from build123d import *

# Parameters (mm, degrees)
SKETCH_1_W                  = 40.6
SKETCH_1_H                  = 45
EXTRUDE_1_DEPTH             = 20
HOLE_WIZARD_M2_1_AT_2_COUNT = 2
HOLE_WIZARD_M2_1_AT_2_PITCH = 20


with BuildPart() as part:
    # 草图1 → 凸台-拉伸1 (new body)
    with BuildSketch(Plane(origin=(0, 0, 0), x_dir=(1, 0, 0), z_dir=(0, 1, 0))):
        Rectangle(SKETCH_1_W, SKETCH_1_H)
    extrude(amount=EXTRUDE_1_DEPTH)

    # 草图3 → M2 螺纹孔的螺纹孔钻头1 (revolve, cut)
    with BuildSketch(Plane(origin=(20.3, 10, 10), x_dir=(0, 0, -1), z_dir=(0, 1, 0))):
        Polygon((0, 0), (0, 8.480688495), (0.8, 8), (0.8, 0), align=None)
    hole_wizard_m2_1 = revolve(axis=Axis((26.65, 10, 10), (-1, 0, 0)), mode=Mode.SUBTRACT)

    # M2 螺纹孔的螺纹孔钻头1 at 2: M2 螺纹孔的螺纹孔钻头1 ×2
    with Locations(*[(0, 0, -i * HOLE_WIZARD_M2_1_AT_2_PITCH) for i in range(1, HOLE_WIZARD_M2_1_AT_2_COUNT)]):
        add(hole_wizard_m2_1, mode=Mode.SUBTRACT)

    # 镜向1: M2 螺纹孔的螺纹孔钻头1 across plane
    add(hole_wizard_m2_1.mirror(Plane(origin=(0, 0, 0), x_dir=(0, 0, 1), z_dir=(1, 0, 0))), mode=Mode.SUBTRACT)

    # 镜向1 copy 1 sketch → 镜向1 copy 1 (revolve, cut)
    with BuildSketch(Plane(origin=(-20.3, 10, -10), x_dir=(0, 0, -1), z_dir=(0, 1, 0))):
        Polygon((0, 0), (0, -8.480688495), (0.8, -8), (0.8, 0), align=None)
    revolve(axis=Axis((-26.65, 10, -10), (-1, 0, 0)), mode=Mode.SUBTRACT)


solid = part.part
CAD build for the part. Positions are in the model's coordinates, mm. A direction names the side the tool comes from. Round coordinates to 2 decimals unless told otherwise and drop trailing zeros. Return JSON: item names as keys, results as strings.
(1) Tool access for faces 1 (the face through (16.356, 9.207, 10.104)), 2 (the face through (-16.356, 9.207, 10.104)), 3 (the face through (0, 20, 0)): list every direction of +Z, -Z, +X, -X, +Y, -Y with a clear straight run to the whole face (end or side of a thin tool).
Answer key:
{"face 1": "+X", "face 2": "-X", "face 3": "+Z, -Z, +X, -X, +Y"}
(2) Wall check: probe 1 along Z at (x, y) = (-17, 10); probe 2 along Y at (x, z) = (17, 10). Give the ranges that are in metal, low to high. Write a range as from..to.
Answer key:
{"probe 1": "z = -22.5..-10.8, -9.2..9.2, 10.8..22.5", "probe 2": "y = 0..9.2, 10.8..20"}
(3) Pull direction Z, two halves, no side cores. Call faces 4 (the face through (0, 10, -22.5)), 5 (the face through (11.903, 9.862, -9.982)), 6 (the face through (-20.3, 10, 0)), 7 (the face through (0, 10, 22.5)): +Z half, -Z half, draft (parallel to the pull), parting line (faces both ways), or undercut.
Answer key:
{"face 4": "-Z half", "face 5": "undercut", "face 6": "draft", "face 7": "+Z half"}
(4) Pin check, flat tip, straight feed: pin 1 Ø1 at (x, z) = (3.5, 2.5) entering from -Y. Stop position of the tip, or through.
Answer key:
{"pin 1": "stops at y = 0"}
